Geometry: final body of the model. Coordinates: model frame, mm. Coordinates: 2 decimals unless noted, no trailing zeros. Write each loop counter-clockwise with the first axis right and the second up, starting at its lowest first coordinate (ties: lowest second). Pieces come first, ordered by that corner, then holes. Notation, with made-up numbers: (-12, -29) -> (23, -29) arc R6 ccw to (23, -19) -> close; hole circle Ø3 at (31.5, -20). An arc over 180 degrees is marked (long way). Answer as a JSON object with one key per item and string values. Group by question number.
Autodesk Inventor part; units mm, degrees
ref_plane "YZ Plane" through (0, 0, 0) normal (1, 0, 0) x (0, 1, 0)
ref_plane "XZ Plane" through (0, 0, 0) normal (0, 1, 0) x (-1, 0, 0)
ref_plane "XY Plane" through (0, 0, 0) normal (0, 0, 1) x (1, 0, 0)
sketch "Sketch1" plane through (0, 0, 0) normal (0, 0, 1) x (1, 0, 0)
  circle A0 centre (0, 0) radius 2.413
  dimension "d0" = 4.826
extrude "Extrusion1" add sketch "Sketch1" along normal blind 50.8
sketch "Sketch2" plane through (0, 0, 0) normal (0, 1, 0) x (-1, 0, 0)
  line L0 (0, 0) -> (0, -2.5654)
  line L1 (0, 0) -> (4.3239, 0)
  line L2 (0, -2.5654) -> (2.032, -2.5654)
  line L3 (4.3239, 0) -> (4.3239, 3.8864) construction
  arc A0 (4.5568, -0.3781) -> (4.3239, 0) centre (4.3239, -0.2608) ccw
  arc A1 (2.032, -2.5654) -> (4.5568, -0.3781) centre (0.6382, 1.5944) ccw
  line L4 (4.5847, 0.6553) -> (4.5847, -0.2608) construction
  dimension "d3" = 2.5654
  dimension "d6" = 2.032
  dimension "d12" = 4.5847
revolve "Revolution1" add sketch "Sketch2" angle 360 about axis through (0, 0, 0) along (0, 0, -1)
sketch "Sketch3" plane through (0, 0, -2.5654) normal (0, 0, -1) x (-1, 0, 0)
  circle A0 centre (0, 0) radius 2.032
  line L0 (-0.9165, 1.5875) -> (0.9165, 1.5875)
  line L1 (0.9165, 1.5875) -> (1.8331, 0)
  line L2 (1.8331, 0) -> (0.9165, -1.5875)
  line L3 (0.9165, -1.5875) -> (-0.9165, -1.5875)
  line L4 (-0.9165, -1.5875) -> (-1.8331, 0)
  line L5 (-1.8331, 0) -> (-0.9165, 1.5875)
  dimension "d8" = 3.175
extrude "Extrusion2" cut sketch "Sketch3" against normal blind 1.5875 contours L0 L1 L2 L3 L4 L5
chamfer "Chamfer1" distance 0.508 angle 45 1 edges at (-2.413, 0, 50.8)
thread "Thread2"
properties part number "10-32 x625 button head" material "Steel"
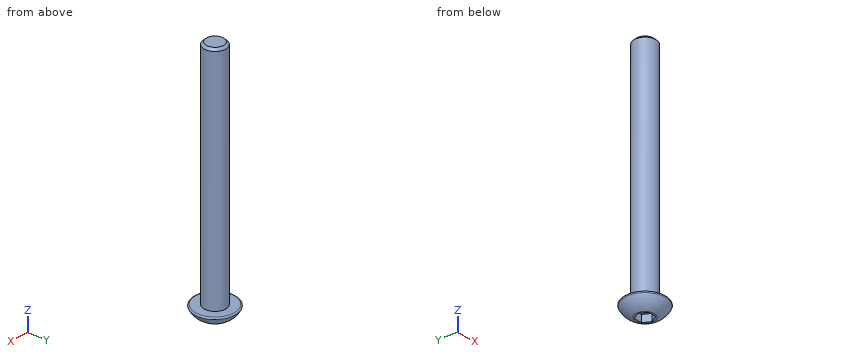
Item 1: Section A-A on z = 39. Output: boundary loops of the cut face in (x, y).
Item 2: Ray query, L1, parallel to Z at x = 0, y = -0.75; L2, parallel to Y at x = 0, z = 11.5; L3, parallel to Z at x = -1.5, y = 3.5. Return the intervals inside material, ascending. Write a range as [from, to].
Item 3: Contact query for flat-ended pins moving along their axis: pin 1 (5 mm diameter, centred on x = -0.5, z = 17, fed in from -Y); pin 2 (1 mm diameter, centred on x = -1, z = 21, fed in from +Y); pin 3 (4 mm diameter, centred on x = 3.5, z = 30.5, fed in from +Y). Output: stop coordinate, or through.
Answer sheet:
{
 "1": {"outline": "circle Ø4.83 at (0, 0)"},
 "2": {"L1": "z = [-0.98, 50.8]", "L2": "y = [-2.41, 2.41]", "L3": "z = [-1.44, 0]"},
 "3": {"pin 1": "stops at y = -2.41", "pin 2": "stops at y = 2.36", "pin 3": "stops at y = 1.89"}
}
